For this review, take the finished solid that the model builds, in its own axes (mm). A direction names the side the tool comes from. Coordinates: 2 decimals unless noted, no trailing zeros. Write each loop counter-clockwise with the first axis right and the second up, starting at its lowest first coordinate (ties: lowest second). Pieces come first, ordered by that corner, then holes.
1) We need section A-A on x = -6.75. Write out the cut boundary in (y, z), then the cut area to 3 significant figures.
2) We need section C-C on x = -10.75. Write out the cut boundary in (y, z).
3) We need section D-D on z = 13.5. Write out the cut boundary in (x, y), then the cut area to 3 significant figures.
4) To check wall thickness, follow line 1 along Y through (x, z) = (4.5, -3); line 2 along Y through (x, z) = (-13.5, -4); line 3 along X through (y, z) = (20, -11). State the ranges of each line that lie inside material, in increasing order.
5) We need section B-B on z = -10. Write out the cut boundary in (x, y).
6) Mouldability with a two-part tool opening along Y and no side actions: class faces 6 (the face through (0, 0, 0)), 7 (the face through (9.246, 50.189, 8.056)), 8 (the face through (-15, 31, 0)) as pulls with the +Y half, pulls with the -Y half, needs draft (parallel to the pull), parting line crosses it, or undercut.
7) Insertion check: P1, Ø3, axis at x = -9, z = -5, coming from the +Y side; P2, Ø15, axis at y = 9, z = 3, coming from the -X side; P3, Ø15, axis at y = 11, z = -4.5, coming from the +X side; P4, Ø2, axis at x = 3.5, z = -6.5, coming from the -Y side. Each pin has a flat end and moves straight along its axis. Give the tip position at first contact, or say it passes through.
8) For faces 1 (the face through (8, 8, 0)), 2 (the face through (-14.628, 15.853, -0.211)), 3 (the face through (7.5, 8, 0)), 4 (the face through (9, 52, 0)), 5 (the face through (-14.5, 31, 0)), list the 3-axis set-ups (+Z, -Z, +X, -X, +Y, -Y) from which the entire face can be reached by the end or side of a thin tool; tool diameter is ignored.
from build123d import *

# Parameters (mm, degrees)
SKETCH1_W                    = 15
SKETCH1_H                    = 30.181487224
BASE_FLANGE2_DEPTH           = 0.5
EDGE_FLANGE1_STRIP_W         = 3.4732
EDGE_FLANGE1_STRIP_H         = 0.5
EDGE_FLANGE1_STRIP_CUT_DEPTH = 30.181487223
EDGE_FLANGE1_DEPTH           = 30.181487223
EDGE_FLANGE2_STRIP_W         = 3.4732
EDGE_FLANGE2_STRIP_H         = 0.5
EDGE_FLANGE2_STRIP_CUT_DEPTH = 30.181487223
EDGE_FLANGE2_DEPTH           = 30.181487223
EDGE_FLANGE6_STRIP_W         = 3.4732
EDGE_FLANGE6_STRIP_H         = 0.5
EDGE_FLANGE6_STRIP_CUT_DEPTH = 30.181487223
EDGE_FLANGE6_DEPTH           = 30.181487223
EDGE_FLANGE7_STRIP_W         = 3.4732
EDGE_FLANGE7_STRIP_H         = 0.5
EDGE_FLANGE7_STRIP_CUT_DEPTH = 30.181487223
EDGE_FLANGE7_DEPTH           = 30.181487223
EDGE_FLANGE8_STRIP_W         = 3.4732
EDGE_FLANGE8_STRIP_H         = 0.5
EDGE_FLANGE8_STRIP_CUT_DEPTH = 30.181487223
EDGE_FLANGE8_DEPTH           = 30.181487223
SKETCH58_R                   = 2
CUT_EXTRUDE1_DEPTH           = 64.437315854


# Sheet-metal steps are written as plain solids
with BuildPart() as part:
    # Sketch1 → Base-Flange2 (new body)
    with BuildSketch(Plane(origin=(0, 0, 0), x_dir=(1, 0, 0), z_dir=(0, 1, 0))):
        Rectangle(SKETCH1_W, SKETCH1_H)
    extrude(amount=BASE_FLANGE2_DEPTH)

    # Edge-Flange1 strip (across the edge) → Edge-Flange1 strip cut (cut)
    with BuildSketch(Plane(origin=(7.5, 0.5, 15.090743612), x_dir=(-1, 0, 0), z_dir=(0, 0, -1))):
        with Locations((-1, -0.25)):
            Rectangle(EDGE_FLANGE1_STRIP_W, EDGE_FLANGE1_STRIP_H)
    extrude(amount=EDGE_FLANGE1_STRIP_CUT_DEPTH, mode=Mode.SUBTRACT)

    # Edge-Flange1 section (across the edge) → Edge-Flange1 (add)
    with BuildSketch(Plane(origin=(7.5, 0.5, 15.090743612), x_dir=(-1, 0, 0), z_dir=(0, 0, -1))):
        with BuildLine():
            Line((-0.5, 0.7366), (-0.5, 15))
            Line((-0.5, 15), (0, 15))
            Line((0, 15), (0, 0.7366))
            ThreePointArc((0, 0.7366), (0.215745145, 0.215745145), (0.7366, 0))
            Line((0.7366, 0), (0.7366, -0.5))
            ThreePointArc((0.7366, -0.5), (-0.137808246, -0.137808246), (-0.5, 0.7366))
        make_face()
    extrude(amount=EDGE_FLANGE1_DEPTH)

    # Edge-Flange2 strip (across the edge) → Edge-Flange2 strip cut (cut)
    with BuildSketch(Plane(origin=(7.5, 15.5, 15.090743612), x_dir=(0, -1, 0), z_dir=(0, 0, -1))):
        with Locations((-1, -0.25)):
            Rectangle(EDGE_FLANGE2_STRIP_W, EDGE_FLANGE2_STRIP_H)
    extrude(amount=EDGE_FLANGE2_STRIP_CUT_DEPTH, mode=Mode.SUBTRACT)

    # Edge-Flange2 section (across the edge) → Edge-Flange2 (add)
    with BuildSketch(Plane(origin=(7.5, 15.5, 15.090743612), x_dir=(0, -1, 0), z_dir=(0, 0, -1))):
        with BuildLine():
            Line((-0.5, 0.7366), (-0.5, 22))
            Line((-0.5, 22), (0, 22))
            Line((0, 22), (0, 0.7366))
            ThreePointArc((0, 0.7366), (0.215745145, 0.215745145), (0.7366, 0))
            Line((0.7366, 0), (0.7366, -0.5))
            ThreePointArc((0.7366, -0.5), (-0.137808246, -0.137808246), (-0.5, 0.7366))
        make_face()
    extrude(amount=EDGE_FLANGE2_DEPTH)

    # Edge-Flange6 strip (across the edge) → Edge-Flange6 strip cut (cut)
    with BuildSketch(Plane(origin=(-14.5, 16, -15.090743612), x_dir=(1, 0, 0), z_dir=(0, 0, 1))):
        with Locations((-1, -0.25)):
            Rectangle(EDGE_FLANGE6_STRIP_W, EDGE_FLANGE6_STRIP_H)
    extrude(amount=EDGE_FLANGE6_STRIP_CUT_DEPTH, mode=Mode.SUBTRACT)

    # Edge-Flange6 section (across the edge) → Edge-Flange6 (add)
    with BuildSketch(Plane(origin=(-14.5, 16, -15.090743612), x_dir=(1, 0, 0), z_dir=(0, 0, 1))):
        with BuildLine():
            Line((-0.5, 0.7366), (-0.5, 30.25))
            Line((-0.5, 30.25), (0, 30.25))
            Line((0, 30.25), (0, 0.7366))
            ThreePointArc((0, 0.7366), (0.215745145, 0.215745145), (0.7366, 0))
            Line((0.7366, 0), (0.7366, -0.5))
            ThreePointArc((0.7366, -0.5), (-0.137808246, -0.137808246), (-0.5, 0.7366))
        make_face()
    extrude(amount=EDGE_FLANGE6_DEPTH)

    # Edge-Flange7 strip (across the edge) → Edge-Flange7 strip cut (cut)
    with BuildSketch(Plane(origin=(-14.5, 46.25, -15.090743612), x_dir=(0, -1, 0), z_dir=(0, 0, 1))):
        with Locations((-1, -0.25)):
            Rectangle(EDGE_FLANGE7_STRIP_W, EDGE_FLANGE7_STRIP_H)
    extrude(amount=EDGE_FLANGE7_STRIP_CUT_DEPTH, mode=Mode.SUBTRACT)

    # Edge-Flange7 section (across the edge) → Edge-Flange7 (add)
    with BuildSketch(Plane(origin=(-14.5, 46.25, -15.090743612), x_dir=(0, -1, 0), z_dir=(0, 0, 1))):
        with BuildLine():
            Line((-0.5, 0.7366), (-0.5, 23.5))
            Line((-0.5, 23.5), (0, 23.5))
            Line((0, 23.5), (0, 0.7366))
            ThreePointArc((0, 0.7366), (0.215745145, 0.215745145), (0.7366, 0))
            Line((0.7366, 0), (0.7366, -0.5))
            ThreePointArc((0.7366, -0.5), (-0.137808246, -0.137808246), (-0.5, 0.7366))
        make_face()
    extrude(amount=EDGE_FLANGE7_DEPTH)

    # Edge-Flange8 strip (across the edge) → Edge-Flange8 strip cut (cut)
    with BuildSketch(Plane(origin=(9, 46.75, 15.090743612), x_dir=(-1, 0, 0), z_dir=(0, 0, -1))):
        with Locations((-1, -0.25)):
            Rectangle(EDGE_FLANGE8_STRIP_W, EDGE_FLANGE8_STRIP_H)
    extrude(amount=EDGE_FLANGE8_STRIP_CUT_DEPTH, mode=Mode.SUBTRACT)

    # Edge-Flange8 section (across the edge) → Edge-Flange8 (add)
    with BuildSketch(Plane(origin=(9, 46.75, 15.090743612), x_dir=(-1, 0, 0), z_dir=(0, 0, -1))):
        with BuildLine():
            Line((-0.5, 0.7366), (-0.5, 10))
            Line((-0.5, 10), (0, 10))
            Line((0, 10), (0, 0.7366))
            ThreePointArc((0, 0.7366), (0.215745145, 0.215745145), (0.7366, 0))
            Line((0.7366, 0), (0.7366, -0.5))
            ThreePointArc((0.7366, -0.5), (-0.137808246, -0.137808246), (-0.5, 0.7366))
        make_face()
    extrude(amount=EDGE_FLANGE8_DEPTH)

    # Sketch58 → Cut-Extrude1 (cut, through all)
    with BuildSketch(Plane.ZY.offset(-9)):
        with Locations(Location((8.82216851, 52.036798661, 0), (0, 0, 270))):
            Circle(SKETCH58_R)
        with Locations(Location((-8.82216851, 52.036798661, 0), (0, 0, 90))):
            Circle(SKETCH58_R)
    extrude(amount=-CUT_EXTRUDE1_DEPTH, mode=Mode.SUBTRACT)


solid = part.part
Result:
1. outline: (0, -15.09) - (0.5, -15.09) - (0.5, 15.09) - (0, 15.09) - close; (15.5, -15.09) - (16, -15.09) - (16, 15.09) - (15.5, 15.09) - close; (46.25, -15.09) - (46.75, -15.09) - (46.75, 15.09) - (46.25, 15.09) - close
1. area: 45.3 mm2
2. outline: (15.5, -15.09) - (16, -15.09) - (16, 15.09) - (15.5, 15.09) - close; (46.25, -15.09) - (46.75, -15.09) - (46.75, 15.09) - (46.25, 15.09) - close
3. outline: (-15, 16.74) arc R1.24 ccw to (-13.76, 15.5) - (6.76, 15.5) arc R0.74 cw to (7.5, 14.76) - (7.5, 1.24) arc R0.74 cw to (6.76, 0.5) - (-7.5, 0.5) - (-7.5, 0) - (6.76, 0) arc R1.24 ccw to (8, 1.24) - (8, 14.76) arc R1.24 ccw to (6.76, 16) - (-13.76, 16) arc R0.74 cw to (-14.5, 16.74) - (-14.5, 45.51) arc R0.74 cw to (-13.76, 46.25) - (8.26, 46.25) arc R1.24 ccw to (9.5, 47.49) - (9.5, 56.75) - (9, 56.75) - (9, 47.49) arc R0.74 cw to (8.26, 46.75) - (-13.76, 46.75) arc R1.24 ccw to (-15, 45.51) - close
3. area: 58.1 mm2
4. line 1: y = 0 to 0.5, 15.5 to 16, 46.25 to 46.75
4. line 2: y = 15.5 to 16, 46.25 to 46.75
4. line 3: x = -15 to -14.5
5. outline: (-15, 16.74) arc R1.24 ccw to (-13.76, 15.5) - (6.76, 15.5) arc R0.74 cw to (7.5, 14.76) - (7.5, 1.24) arc R0.74 cw to (6.76, 0.5) - (-7.5, 0.5) - (-7.5, 0) - (6.76, 0) arc R1.24 ccw to (8, 1.24) - (8, 14.76) arc R1.24 ccw to (6.76, 16) - (-13.76, 16) arc R0.74 cw to (-14.5, 16.74) - (-14.5, 45.51) arc R0.74 cw to (-13.76, 46.25) - (8.26, 46.25) arc R1.24 ccw to (9.5, 47.49) - (9.5, 50.42) - (9, 50.42) - (9, 47.49) arc R0.74 cw to (8.26, 46.75) - (-13.76, 46.75) arc R1.24 ccw to (-15, 45.51) - close; (9, 53.65) - (9.5, 53.65) - (9.5, 56.75) - (9, 56.75) - close
6. face 6: pulls with the -Y half
6. face 7: undercut
6. face 8: needs draft
7. P1: stops at y = 46.75
7. P2: stops at x = -14.98
7. P3: stops at x = 8
7. P4: stops at y = 0
8. face 1: +Z, -Z, +X, -Y
8. face 2: +Z, -Z, -X, -Y
8. face 3: +Z, -Z, -X
8. face 4: +Z, -Z, -X, +Y
8. face 5: +Z, -Z, +X
